Geometry: see drawing. Coordinates: mm, zero at the bounding-box minimum. Coordinates: 2 decimals unless noted, no trailing zeros. Order: outer loops, then holes, each group sorted by start corner. A loop starts at its lowest first (then second) coordinate and runs counter-clockwise, first axis right, second up. Notation, with made-up numbers: (37, 59) -> (90, 59) arc R28 cw to (90, 82) -> close; hole circle Ø6 at (-37.75, 61). An arc over 180 degrees is marked (long way). Write each question's results on one line, items separated by ' | '.
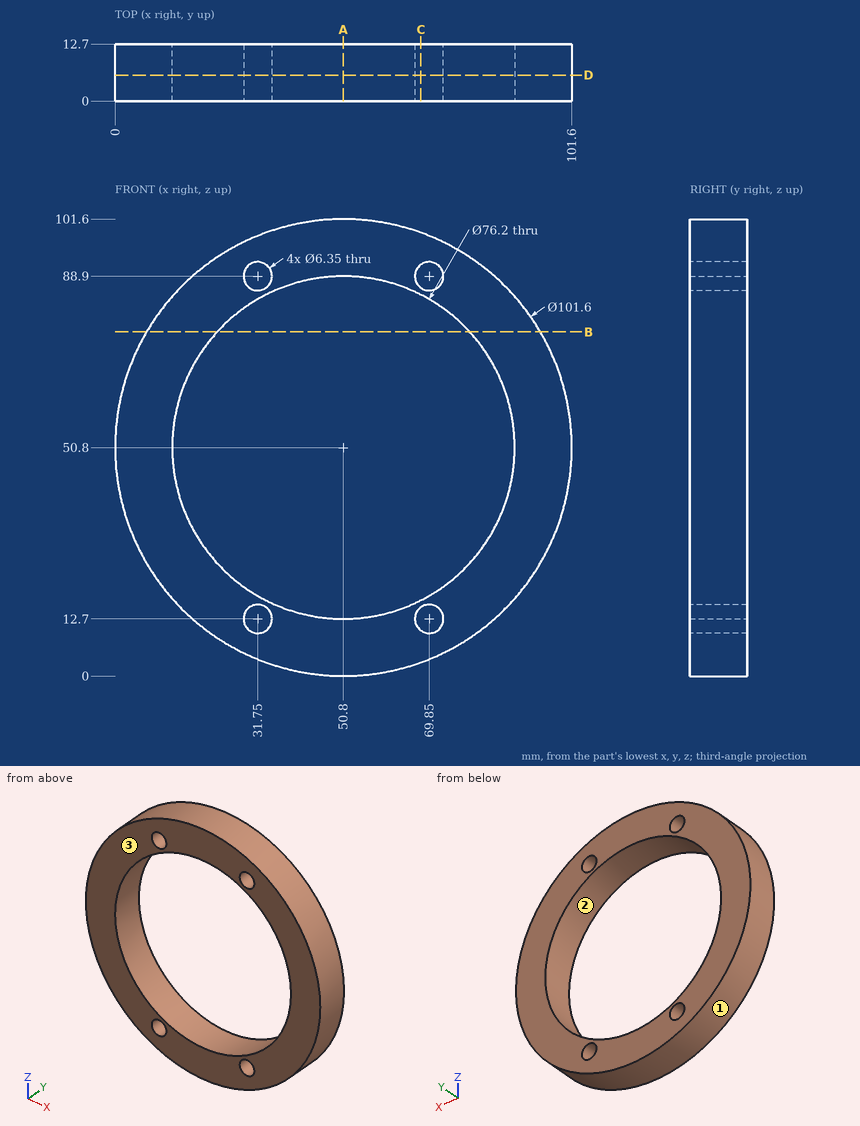
(1) Cut plane C-C, the plane x = 68. Return loops of the section in (y, z).
Return value:
outline: (0, 3) -> (12.7, 3) -> (12.7, 10.12) -> (0, 10.12) -> close; (0, 15.28) -> (12.7, 15.28) -> (12.7, 16.8) -> (0, 16.8) -> close; (0, 84.8) -> (12.7, 84.8) -> (12.7, 86.32) -> (0, 86.32) -> close; (0, 91.48) -> (12.7, 91.48) -> (12.7, 98.6) -> (0, 98.6) -> close
(2) Line query: line 1 along Z through (x, y) = (31.75, 5.25) (3 decimals); line 2 along Z through (x, y) = (32, 6.5); line 3 along Z through (x, y) = (50.8, 6.5). Output: solid intervals per line, ascending. Write a range as from..to.
Return value:
line 1: 3.707..9.525, 15.875..17.804, 83.796..85.725, 92.075..97.893 | line 2: 3.61..9.53, 15.87..17.66, 83.94..85.73, 92.07..97.99 | line 3: 0..12.7, 88.9..101.6
(3) Pin query (flat end, axial travel): P1, Ø4, axis at x = 91, y = 10, coming from the -Z side; P2, Ø2, axis at y = 2, z = 68.5, coming from the -X side; P3, Ø6, axis at x = 20, y = 7.5, coming from the +Z side. Return the tip coordinate at first contact, or that it passes through.
Return value:
P1: z = 17.31 | P2: x = 2.82 | P3: z = 93.32
(4) Mould query, pull axis Z, two halves, no side actions, for the marked faces 1, 2 and 3. Classes: +Z half, -Z half, draft (parallel to the pull), parting line (faces both ways), or undercut.
Return value:
face 1: parting line | face 2: undercut | face 3: draft
(5) Cut plane D-D, the plane y = 5.75. Return loops of the section in (x, z) (3 decimals).
Return value:
outline: circle Ø101.6 at (50.8, 50.8); hole circle Ø76.2 at (50.8, 50.8); hole circle Ø6.35 at (31.75, 12.7); hole circle Ø6.35 at (31.75, 88.9); hole circle Ø6.35 at (69.85, 12.7); hole circle Ø6.35 at (69.85, 88.9)
(6) Cut plane B-B, the plane z = 76.5. Return loops of the section in (x, y).
Return value:
outline: (6.98, 0) -> (22.67, 0) -> (22.67, 12.7) -> (6.98, 12.7) -> close; (78.93, 0) -> (94.62, 0) -> (94.62, 12.7) -> (78.93, 12.7) -> close
(7) Cut plane A-A, the plane x = 50.8. Return loops of the section in (y, z).
Return value:
outline: (0, 0) -> (12.7, 0) -> (12.7, 12.7) -> (0, 12.7) -> close; (0, 88.9) -> (12.7, 88.9) -> (12.7, 101.6) -> (0, 101.6) -> close
